Read the model definition and answer for the solid it produces. Units are mm, in the model's axes. Face numbers are marked on the shaded views. A direction names the side the tool comes from. Round coordinates to 2 decimals unless told otherwise and drop trailing zeros. Write each loop counter-clockwise with the first axis right and the second up, starting at its lowest first coordinate (ties: lowest second). Pieces come first, ordered by that corner, then holes. Notation, with made-up numbers: (4, 55) - (17, 55) arc R28 ccw to (17, 81) - close; hole circle Ø4 at (43.5, 19). An arc over 180 degrees is marked (long way). One line per item, written item: value. Start each with the question number.
(1) A cutting plane is placed at C-C, the plane x = 10. Determine the outline of the cut face in (y, z).
(2) A cutting plane is placed at A-A, the plane z = -21. Determine the outline of the cut face in (x, y).
(3) A cutting plane is placed at D-D, the plane y = 17.5. Determine the outline of the cut face in (x, z), plus the area to 3 significant figures.
(4) For the marked faces 1, 2 and 3, determine the directions among +Z, -Z, +X, -X, +Y, -Y from which every point of the face is accessible in a straight line to the end or side of a thin tool.
(5) Find the intervals of material crossed by L1, parallel to X at y = 7, z = -21; L2, parallel to Y at x = 23, z = 6; L3, parallel to X at y = 11, z = -22, in increasing order.
(6) Flat-ended cylindrical pins translate along their axes: pin 1 Ø9 at (x, y) = (-6.5, 20.5) entering from -Z; pin 2 Ø3.5 at (x, z) = (-39.5, 21) entering from -Y; pin 3 Ø3.5 at (x, z) = (-39.5, -21) entering from +Y; pin 4 Ø6.5 at (x, y) = (-6.5, 20.5) entering from +Z. Find the tip coordinate at first contact, or state that the pin passes through.
(7) A cutting plane is placed at B-B, the plane x = 39.5. Determine the outline of the cut face in (y, z), plus the area to 3 significant figures.
from build123d import *

# Parameters (mm, degrees)
SKETCH_1_W      = 87
SKETCH_1_H      = 50
SKETCH_1_R      = 1.6
EXTRUDE_1_DEPTH = 15
SKETCH_2_W      = 36
SKETCH_2_H      = 36
EXTRUDE_2_DEPTH = 8


with BuildPart() as part:
    # 草图1 → 凸台-拉伸1 (new body)
    with BuildSketch(Plane(origin=(0, 0, 0), x_dir=(1, 0, 0), z_dir=(0, 1, 0))):
        Rectangle(SKETCH_1_W, SKETCH_1_H)
        with Locations(Location((-39.5, 21, 0), (0, 0, 270))):
            Circle(SKETCH_1_R, mode=Mode.SUBTRACT)
        with Locations(Location((39.5, 21, 0), (0, 0, 90))):
            Circle(SKETCH_1_R, mode=Mode.SUBTRACT)
        with Locations(Location((39.5, -21, 0), (0, 0, 270))):
            Circle(SKETCH_1_R, mode=Mode.SUBTRACT)
        with Locations(Location((-39.5, -21, 0), (0, 0, 90))):
            Circle(SKETCH_1_R, mode=Mode.SUBTRACT)
    extrude(amount=EXTRUDE_1_DEPTH)

    # 草图2 → 凸台-拉伸2 (add)
    with BuildSketch(Plane(origin=(0, 15, 0), x_dir=(1, 0, 0), z_dir=(0, 1, 0))):
        with Locations((-1.022681739, 4.732356083)):
            Rectangle(SKETCH_2_W, SKETCH_2_H)
    extrude(amount=EXTRUDE_2_DEPTH)


solid = part.part
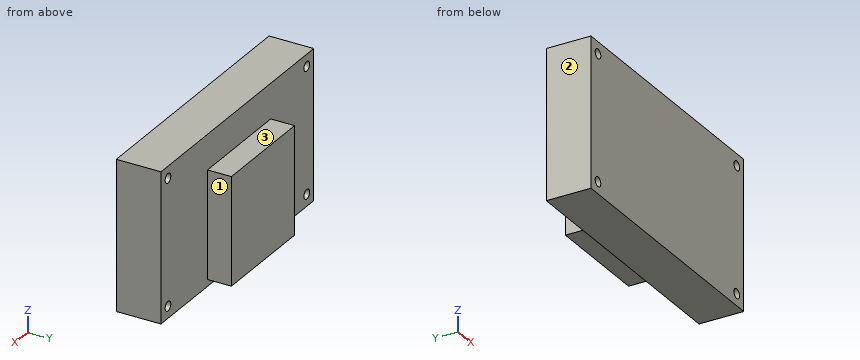
Here are the results:
1. outline: (0, -25) - (15, -25) - (15, -22.73) - (23, -22.73) - (23, 13.27) - (15, 13.27) - (15, 25) - (0, 25) - close
2. outline: (-43.5, 0) - (-41.1, 0) - (-41.1, 15) - (-43.5, 15) - close; (-37.9, 0) - (37.9, 0) - (37.9, 15) - (16.98, 15) - (16.98, 23) - (-19.02, 23) - (-19.02, 15) - (-37.9, 15) - close; (41.1, 0) - (43.5, 0) - (43.5, 15) - (41.1, 15) - close
3. outline: (-19.02, -22.73) - (16.98, -22.73) - (16.98, 13.27) - (-19.02, 13.27) - close
3. area: 1,300 mm²
4. face 1: +Z, -Z, +X, +Y
4. face 2: +Z, -Z, -X, +Y, -Y
4. face 3: +Z, +X, -X, +Y
5. L1: -43.5 to -41.1, -37.9 to 37.9, 41.1 to 43.5
5. L2: 0 to 15
5. L3: -43.5 to -40.75, -38.25 to 38.25, 40.75 to 43.5
6. pin 1: z = -22.73
6. pin 2: y = 0
6. pin 3: y = 15
6. pin 4: z = 13.27
7. outline: (0, -25) - (15, -25) - (15, -22.6) - (0, -22.6) - close; (0, -19.4) - (15, -19.4) - (15, 19.4) - (0, 19.4) - close; (0, 22.6) - (15, 22.6) - (15, 25) - (0, 25) - close
7. area: 654 mm²
